Input: part model. Units: mm. Frame: model coordinates. Face numbers are marked on the shaded views. A direction names the side the tool comes from. Coordinates: 2 decimals unless noted, no trailing zeros. Loops run counter-clockwise (first coordinate to the right, second up) from the corner with the lowest first, then second, coordinate; pieces in that order, holes last.
(1) Section D-D, the plane y = 54.5. Return loops of the section in (x, z).
(2) Section C-C, the plane x = 41. Return loops of the section in (y, z), then the cut area to 3 significant figures.
(3) Line query: L1, parallel to X at y = 47, z = 1.5; L2, parallel to Z at x = 39.5, y = 40.5; L3, parallel to Y at x = 37.5, z = 4.25. Output: solid intervals per line, ascending.
(4) Contact query for flat-ended pins moving along their axis: P1, Ø5, axis at x = 24.5, z = 8, coming from the -Y side; P2, Ø3.5, axis at x = 47.43, y = 28.6, coming from the -Z side. Output: stop coordinate, or through.
(5) Set-up query: the marked faces 4 and 5. Return all of +Z, -Z, +X, -X, +Y, -Y with unobstructed straight access to the full face (end or side cutting, diameter ignored); none if empty.
(6) Section A-A, the plane y = 25.5. Return loops of the section in (x, z).
(7) Section B-B, the plane z = 2. Return loops of the section in (x, y), then the cut area to 3 significant figures.
(8) Mould query, pull axis Z, two halves, no side actions, for the marked faces 1, 2 and 3. Classes: released by +Z, released by -Z, zero draft, split by the parting line, or undercut.
```python
from build123d import *

# Parameters (mm, degrees)
SKETCH001_AS_DRAWN_W                      = 35
SKETCH001_AS_DRAWN_H                      = 4.5
EXTRUDE001_DEPTH                          = 15
EXTRUDE001_ONTO_SKETCH001_ROLL_ANGLE      = 90
EXTRUDE001_ONTO_SKETCH001_PLACEMENT_ANGLE = -92.306069
EXTRUDE001_PLACEMENT_ANGLE                = 15
SKETCH002_R                               = 1.94
EXTRUDE002_DEPTH                          = 15
EXTRUDE_DEPTH                             = 13.5


with BuildPart() as extrude001:
    # Sketch001 as drawn → Extrude001 (new)
    with BuildSketch(Plane.XY):
        with Locations((-28.593868, 6.75)):
            Rectangle(SKETCH001_AS_DRAWN_W, SKETCH001_AS_DRAWN_H)
    extrude(amount=-EXTRUDE001_DEPTH)


with BuildPart() as extrude001_1:
    # Extrude001 onto Sketch001 roll: moved
    add(extrude001.part.rotate(Axis((0, 0, 0), (1, 0, 0)), EXTRUDE001_ONTO_SKETCH001_ROLL_ANGLE))


with BuildPart() as extrude001_2:
    # Extrude001 onto Sketch001 placement: moved
    add(extrude001_1.part.moved(Location((24.697887, -0.99459, 0))).rotate(Axis((24.697887, -0.99459, 0), (0, 0, 1)), EXTRUDE001_ONTO_SKETCH001_PLACEMENT_ANGLE))


with BuildPart() as extrude001_3:
    # Extrude001 placement: moved
    add(extrude001_2.part.moved(Location((17.714834, -0.429705, 0))).rotate(Axis((17.714834, -0.429705, 0), (0, 0, 1)), EXTRUDE001_PLACEMENT_ANGLE))


with BuildPart() as extrude002:
    # Sketch002 → Extrude002 (new body)
    with BuildSketch(Plane.XY.offset(13.5)):
        with Locations((36.775076, 43.105323)):
            Circle(SKETCH002_R)
        with Locations((47.431625, 28.598843)):
            Circle(SKETCH002_R)
    extrude(amount=-EXTRUDE002_DEPTH)


with BuildPart() as cut001:
    # Sketch → Extrude (new body)
    with BuildSketch(Plane.XY):
        Polygon((34.239132, 42.01487), (50.255318, 19.660189), (50.255318, 62.160189), (22.716467, 87.104851), (17.308471, 86.162684), (22.590996, 72.123634), (34.239132, 55.865684), align=None)
    extrude(amount=EXTRUDE_DEPTH)

    # Cut: cut Extrude002
    add(extrude002.part, mode=Mode.SUBTRACT)

    # Cut001: cut Extrude001
    add(extrude001_3.part, mode=Mode.SUBTRACT)


solid = cut001.part
```
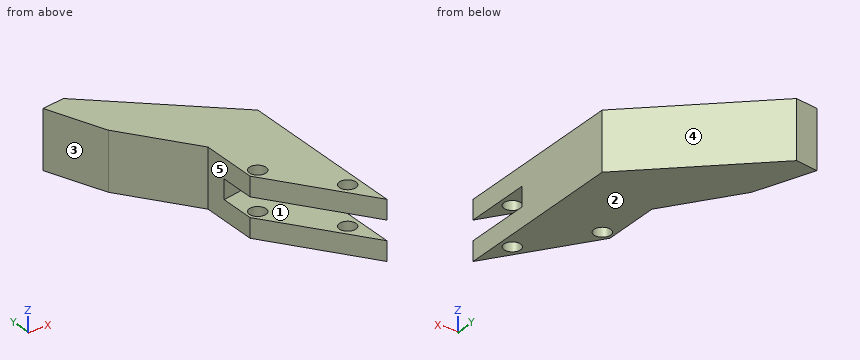
Report:
1. outline: (34.24, 0) - (50.26, 0) - (50.26, 13.5) - (34.24, 13.5) - close
2. outline: (32.58, 0) - (70.54, 0) - (70.54, 13.5) - (32.58, 13.5) - (32.58, 9) - (52.06, 9) - (52.06, 4.5) - (32.58, 4.5) - close
2. area: 425 mm2
3. L1: x = 34.24 to 50.26
3. L2: z = 0 to 4.5, 9 to 13.5
3. L3: y = 37.46 to 41.31, 44.9 to 73.71
4. P1: stops at y = 65.97
4. P2: passes through
5. face 4: +Z, -Z, +X, +Y
5. face 5: +Z, -Z, -X, -Y
6. outline: (46.07, 0) - (50.26, 0) - (50.26, 4.5) - (46.07, 4.5) - close; (46.07, 9) - (50.26, 9) - (50.26, 13.5) - (46.07, 13.5) - close
7. outline: (17.31, 86.16) - (22.59, 72.12) - (34.24, 55.87) - (34.24, 42.01) - (50.26, 19.66) - (50.26, 62.16) - (22.72, 87.1) - close; hole circle Ø3.88 at (36.78, 43.11); hole circle Ø3.88 at (47.43, 28.6)
7. area: 843 mm2
8. face 1: undercut
8. face 2: released by -Z
8. face 3: zero draft
